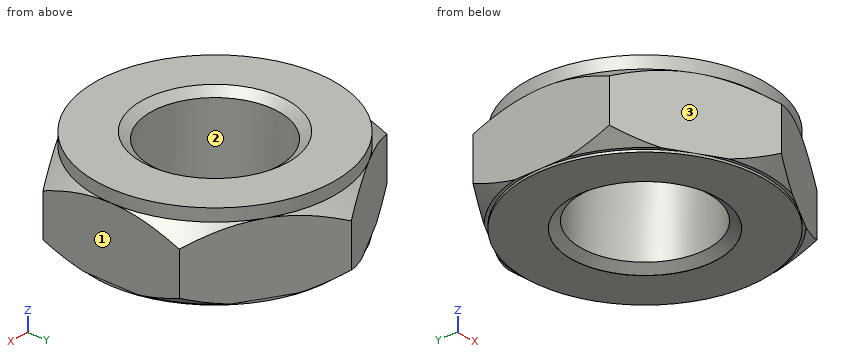
from build123d import *

# Parameters (mm, degrees)
BASENUT_START = -14.605
BASENUTSKE_R  = 11.1125
BASENUT_DEPTH = 14.605
SKETCH4_W     = 0.4064
SKETCH4_H     = 15.892632361


with BuildPart() as part:
    # BaseNutSke → BaseNut (new body)
    with BuildSketch(Plane.XY.offset(BASENUT_START)):
        Polygon((20.6375, 11.91506618), (20.6375, -11.91506618), (0, -23.830132361), (-20.6375, -11.91506618), (-20.6375, 11.91506618), (0, 23.830132361), align=None)
        Circle(BASENUTSKE_R, mode=Mode.SUBTRACT)
    extrude(amount=BASENUT_DEPTH)

    # Sketch4 → Bearing-Face (revolve, cut)
    with BuildSketch(Plane(origin=(0, 0, 0), x_dir=(0, 0, -1), z_dir=(1, 0, 0)), mode=Mode.PRIVATE) as bearing_face_sk:
        with Locations((14.4018, 28.583816181)):
            Rectangle(SKETCH4_W, SKETCH4_H)
        Polygon((0, 20.6375), (-12.7, 20.6375), (-12.7, 36.530132361), (2.54, 36.530132361), (2.54, 23.830132361), align=None)
    revolve(bearing_face_sk.sketch.rotate(Axis((0, 0, 0), (0, 0, -1)), 90), axis=Axis((0, 0, 0), (0, 0, -1)), mode=Mode.SUBTRACT)

    # Sketch3 → Double-Chamfer (revolve, cut)
    with BuildSketch(Plane(origin=(0, 0, 0), x_dir=(0, 0, -1), z_dir=(1, 0, 0)), mode=Mode.PRIVATE) as double_chamfer_sk:
        Polygon((14.605, 20.6375), (12.065, 23.830132361), (12.065, 36.530132361), (27.305, 36.530132361), (27.305, 20.6375), align=None)
        Polygon((4.6736, 36.530132361), (-10.5664, 36.530132361), (-10.5664, 20.6375), (2.1336, 20.6375), (4.6736, 23.830132361), align=None)
    revolve(double_chamfer_sk.sketch.rotate(Axis((0, 0, 0), (0, 0, -1)), 90), axis=Axis((0, 0, 0), (0, 0, -1)), mode=Mode.SUBTRACT)

    # EndChamferSke → EndChamfer (revolve, cut)
    with BuildSketch(Plane(origin=(0, 0, 0), x_dir=(0, 0, -1), z_dir=(1, 0, 0)), mode=Mode.PRIVATE) as endchamfer_sk:
        Polygon((14.5796, 12.7), (13.356862586, 10.95375), (14.6304, 10.95375), (14.6304, 12.7), align=None)
        Polygon((-0.0508, 12.7), (0, 12.7), (1.222737414, 10.95375), (-0.0508, 10.95375), align=None)
    revolve(endchamfer_sk.sketch.rotate(Axis((0, 0, -25.037505729), (0, 0, -1)), 90), axis=Axis((0, 0, -25.037505729), (0, 0, -1)), mode=Mode.SUBTRACT)


solid = part.part
Model file for the job. Use its own axes, mm. Face numbers are marked on the shaded views. Give positions to 0.01 mm unless a question says otherwise; leave off trailing zeros. Order: outer loops, then holes, each group sorted by start corner. A loop starts at its lowest first (then second) coordinate and runs counter-clockwise, first axis right, second up. Notation, with made-up numbers: (26.25, 83) - (83.25, 83) arc R28 cw to (83.25, 107) - close; hole circle Ø10 at (46.25, -9.5). An arc over 180 degrees is marked (long way). One line per item, written item: value.
Item 1: Two-plate mould, pull along X, no slides. Class the marked faces 1, 2 and 3: released by +X, released by -X, zero draft, split by the parting line, or undercut.
Response values:
face 1: released by +X
face 2: undercut
face 3: released by -X
Item 2: Slice it at A-A (z = -8.25). List the corners of the cut face in (x, y) (1 decimal).
Response values:
outline: (-20.6, -11.9) - (0, -23.8) - (20.6, -11.9) - (20.6, 11.9) - (0, 23.8) - (-20.6, 11.9) - close; hole circle Ø22.2 at (0, 0)
Item 3: Wall check: line 1 (X direction, y = -2, z = -2.75); line 2 (X direction, y = 8.5, z = -3.75); line 3 (Y direction, x = 0, z = -14.55). Give the ranges that are in metal, low to high.
Response values:
line 1: -20.64 to -10.93, 10.93 to 20.64
line 2: -20.64 to -7.16, 7.16 to 20.64
line 3: -20.64 to -12.66, 12.66 to 20.64
Item 4: Pin check, flat tips, straight feed: pin 1 Ø15 at (x, y) = (0, 0) entering from +Z; pin 2 Ø1 at (x, z) = (5, -12) entering from -Y. Stop position of each tip, or through.
Response values:
pin 1: through
pin 2: y = -21.23
